from build123d import *

# Parameters (mm, degrees)
EXTRUDE_2_DEPTH     = 5
EXTRUDE_2_2_DEPTH   = 5
EXTRUDE_3_DEPTH     = 50
EXTRUDE_4_DEPTH     = 10
CUT_EXTRUDE_1_DEPTH = 7.5
SKETCH_9_R          = 1.25
CUT_EXTRUDE_3_DEPTH = 20
SKETCH_10_R         = 8
SKETCH_10_R_2       = 1.25
CUT_EXTRUDE_7_DEPTH = 5
SKETCH_1_9_R        = 1.25
EXTRUDE_5_DEPTH     = 45
SKETCH_14_R         = 1.25
CUT_EXTRUDE_8_DEPTH = 14
EXTRUDE_6_DEPTH     = 15


# Read off the part's stored shape, not the designer's step: the extrude step
with BuildPart() as part:
    # Sketch 1 → Extrude 2 (new body)
    with BuildSketch(Plane(origin=(0, 0, 0), x_dir=(1, 0, 0), z_dir=(0, 1, 0))):
        with BuildLine():
            Line((56.548408352, 75.246242124), (-83.374180902, 75.246242124))
            Line((-83.374180902, 75.246242124), (-83.374180902, 65.246242124))
            ThreePointArc((-83.374180902, 65.246242124), (-84.838646996, 61.710708218), (-88.374180902, 60.246242124))
            Line((-88.374180902, 60.246242124), (-98.374180902, 60.246242124))
            Line((-98.374180902, 60.246242124), (-98.374180902, -54.753757876))
            Line((-98.374180902, -54.753757876), (-88.374180902, -54.753757876))
            ThreePointArc((-88.374180902, -54.753757876), (-84.838646996, -56.21822397), (-83.374180902, -59.753757876))
            Line((-83.374180902, -59.753757876), (-83.374180902, -69.753757876))
            Line((-83.374180902, -69.753757876), (96.625819098, -69.753757876))
            Line((96.625819098, -69.753757876), (96.625819098, -59.753757876))
            ThreePointArc((96.625819098, -59.753757876), (98.090285193, -56.21822397), (101.625819098, -54.753757876))
            Line((101.625819098, -54.753757876), (111.625819098, -54.753757876))
            Line((111.625819098, -54.753757876), (111.625819098, 14.619924984))
            Line((111.625819098, 14.619924984), (105.067595409, 14.619924984))
            ThreePointArc((105.067595409, 14.619924984), (100.381304866, 17.876743713), (101.799973847, 23.404452606))
            Line((101.799973847, 23.404452606), (106.763929588, 27.690411234))
            Line((106.763929588, 27.690411234), (71.686518841, 68.316728374))
            Line((71.686518841, 68.316728374), (64.816029914, 62.384638559))
            ThreePointArc((64.816029914, 62.384638559), (59.467315828, 61.622843062), (56.548408352, 66.169166182))
            Line((56.548408352, 66.169166182), (56.548408352, 75.246242124))
        make_face()
        Polygon((18.529202454, 9.525154804), (27.612068748, 17.367446554), (47.217798123, -5.33971918), (38.134931829, -13.18201093), align=None, mode=Mode.SUBTRACT)
    extrude(amount=EXTRUDE_2_DEPTH)

    # Sketch 1_6 → Extrude 3 (add)
    with BuildSketch(Plane(origin=(0, 0, 0), x_dir=(1, 0, 0), z_dir=(0, 1, 0))):
        with BuildLine():
            Line((116.625819098, 34.900965901), (116.625819098, -62.253757876))
            ThreePointArc((116.625819098, -62.253757876), (112.964653863, -71.092592641), (104.125819098, -74.753757876))
            Line((104.125819098, -74.753757876), (-90.874180902, -74.753757876))
            ThreePointArc((-90.874180902, -74.753757876), (-99.713015666, -71.092592641), (-103.374180902, -62.253757876))
            Line((-103.374180902, -62.253757876), (-103.374180902, 67.746242124))
            ThreePointArc((-103.374180902, 67.746242124), (-99.713015666, 76.585076889), (-90.874180902, 80.246242124))
            Line((-90.874180902, 80.246242124), (76.449603474, 80.246242124))
            ThreePointArc((76.449603474, 80.246242124), (79.57124226, 79.565726803), (82.126394907, 77.647674468))
            Line((82.126394907, 77.647674468), (114.802610532, 39.802398244))
            ThreePointArc((114.802610532, 39.802398244), (116.155254913, 37.515737807), (116.625819098, 34.900965901))
        make_face()
        with BuildLine():
            ThreePointArc((111.625819098, 19.269608073), (111.155254913, 21.88437998), (109.802610532, 24.171040417))
            Line((109.802610532, 24.171040417), (67.947110848, 72.647674468))
            ThreePointArc((67.947110848, 72.647674468), (65.3919582, 74.565726803), (62.270319414, 75.246242124))
            Line((62.270319414, 75.246242124), (-90.874180902, 75.246242124))
            ThreePointArc((-90.874180902, 75.246242124), (-96.17748176, 73.049542983), (-98.374180902, 67.746242124))
            Line((-98.374180902, 67.746242124), (-98.374180902, -62.253757876))
            ThreePointArc((-98.374180902, -62.253757876), (-96.17748176, -67.557058735), (-90.874180902, -69.753757876))
            Line((-90.874180902, -69.753757876), (104.125819098, -69.753757876))
            ThreePointArc((104.125819098, -69.753757876), (109.429119957, -67.557058735), (111.625819098, -62.253757876))
            Line((111.625819098, -62.253757876), (111.625819098, 19.269608073))
        make_face(mode=Mode.SUBTRACT)
    extrude(amount=EXTRUDE_3_DEPTH)

    # Extrude 4 outline → Extrude 4 (add)
    with BuildSketch(Plane(origin=(0, 0, 0), x_dir=(1, 0, 0), z_dir=(0, 1, 0))):
        Polygon((43.4332705, -8.607340743), (23.827541125, 14.099824991), (22.313730076, 12.792776366), (41.919459451, -9.914389368), align=None)
    extrude(amount=EXTRUDE_4_DEPTH)

    # Sketch 6 → Cut-Extrude 1 (cut)
    with BuildSketch(Plane(origin=(85.459602861, 0, -73.787185323), x_dir=(-0.6535243124977221, 0, -0.7569055244707755), z_dir=(0.7569055244707754, 0, -0.653524312497722))):
        with BuildLine():
            Line((-22.999642003, 24.2), (-22.999642003, 21.9))
            Line((-22.999642003, 21.9), (-16.799642003, 21.9))
            Line((-16.799642003, 21.9), (-16.799642003, 24.2))
            ThreePointArc((-16.799642003, 24.2), (-15.999642003, 25), (-16.799642003, 25.8))
            Line((-16.799642003, 25.8), (-16.799642003, 27.1))
            Line((-16.799642003, 27.1), (-17.799642003, 28.1))
            Line((-17.799642003, 28.1), (-21.999642003, 28.1))
            Line((-21.999642003, 28.1), (-22.999642003, 27.1))
            Line((-22.999642003, 27.1), (-22.999642003, 25.8))
            ThreePointArc((-22.999642003, 25.8), (-23.799642003, 25), (-22.999642003, 24.2))
        make_face()
    extrude(amount=-CUT_EXTRUDE_1_DEPTH, mode=Mode.SUBTRACT)

    # Sketch 9 → Cut-Extrude 3 (cut)
    with BuildSketch(Plane(origin=(79.782811427, 0, -68.885752979), x_dir=(-0.6535243124977224, 0, -0.7569055244707754), z_dir=(0.7569055244707754, 0, -0.6535243124977224))):
        with Locations((-19.899642003, 25)):
            Circle(SKETCH_9_R)
    extrude(amount=-CUT_EXTRUDE_3_DEPTH, mode=Mode.SUBTRACT)

    # Sketch 10 → Cut-Extrude 7 (cut)
    with BuildSketch(Plane.ZY.offset(103.374180902)):
        with Locations((-2.746242124, 25)):
            Circle(SKETCH_10_R)
        with Locations((-59.046242124, 24)):
            Circle(SKETCH_10_R_2)
        with Locations((53.553757876, 24)):
            Circle(SKETCH_10_R_2)
    extrude(amount=-CUT_EXTRUDE_7_DEPTH, mode=Mode.SUBTRACT)

    # Sketch 1_9 → Extrude 5 (add)
    # profile 1 of 5: a face of its own
    with BuildSketch(Plane(origin=(0, 0, 0), x_dir=(1, 0, 0), z_dir=(0, 1, 0))):
        with BuildLine():
            Line((-83.374180902, 75.246242124), (-90.874180902, 75.246242124))
            ThreePointArc((-90.874180902, 75.246242124), (-96.17748176, 73.049542983), (-98.374180902, 67.746242124))
            Line((-98.374180902, 67.746242124), (-98.374180902, 60.246242124))
            Line((-98.374180902, 60.246242124), (-88.374180902, 60.246242124))
            ThreePointArc((-88.374180902, 60.246242124), (-84.838646996, 61.710708218), (-83.374180902, 65.246242124))
            Line((-83.374180902, 65.246242124), (-83.374180902, 75.246242124))
        make_face()
        with Locations(Location((-90.874180902, 67.746242124, 0), (0, 0, 90))):
            Circle(SKETCH_1_9_R, mode=Mode.SUBTRACT)
    # profile 2 of 5: a face of its own
    with BuildSketch(Plane(origin=(0, 0, 0), x_dir=(1, 0, 0), z_dir=(0, 1, 0))):
        with BuildLine():
            Line((-88.374180902, -54.753757876), (-98.374180902, -54.753757876))
            Line((-98.374180902, -54.753757876), (-98.374180902, -62.253757876))
            ThreePointArc((-98.374180902, -62.253757876), (-96.17748176, -67.557058735), (-90.874180902, -69.753757876))
            Line((-90.874180902, -69.753757876), (-83.374180902, -69.753757876))
            Line((-83.374180902, -69.753757876), (-83.374180902, -59.753757876))
            ThreePointArc((-83.374180902, -59.753757876), (-84.838646996, -56.21822397), (-88.374180902, -54.753757876))
        make_face()
        with Locations(Location((-90.874180902, -62.253757876, 0), (0, 0, 90))):
            Circle(SKETCH_1_9_R, mode=Mode.SUBTRACT)
    # profile 3 of 5: a face of its own
    with BuildSketch(Plane(origin=(0, 0, 0), x_dir=(1, 0, 0), z_dir=(0, 1, 0))):
        with BuildLine():
            Line((96.625819098, -59.753757876), (96.625819098, -69.753757876))
            Line((96.625819098, -69.753757876), (104.125819098, -69.753757876))
            ThreePointArc((104.125819098, -69.753757876), (109.429119957, -67.557058735), (111.625819098, -62.253757876))
            Line((111.625819098, -62.253757876), (111.625819098, -54.753757876))
            Line((111.625819098, -54.753757876), (101.625819098, -54.753757876))
            ThreePointArc((101.625819098, -54.753757876), (98.090285193, -56.21822397), (96.625819098, -59.753757876))
        make_face()
        with Locations(Location((104.125819098, -62.253757876, 0), (0, 0, 90))):
            Circle(SKETCH_1_9_R, mode=Mode.SUBTRACT)
    # profile 4 of 5: a face of its own
    with BuildSketch(Plane(origin=(0, 0, 0), x_dir=(1, 0, 0), z_dir=(0, 1, 0))):
        with BuildLine():
            Line((109.802610532, 24.171040417), (106.763929588, 27.690411234))
            Line((106.763929588, 27.690411234), (101.799973847, 23.404452606))
            ThreePointArc((101.799973847, 23.404452606), (100.381304866, 17.876743713), (105.067595409, 14.619924984))
            Line((105.067595409, 14.619924984), (111.625819098, 14.619924984))
            Line((111.625819098, 14.619924984), (111.625819098, 19.269608073))
            ThreePointArc((111.625819098, 19.269608073), (111.155254913, 21.88437998), (109.802610532, 24.171040417))
        make_face()
        with Locations(Location((105.067595409, 19.619924984, 0), (0, 0, 90))):
            Circle(SKETCH_1_9_R, mode=Mode.SUBTRACT)
    # profile 5 of 5: a face of its own
    with BuildSketch(Plane(origin=(0, 0, 0), x_dir=(1, 0, 0), z_dir=(0, 1, 0))):
        with BuildLine():
            Line((62.270319414, 75.246242124), (56.548408352, 75.246242124))
            Line((56.548408352, 75.246242124), (56.548408352, 66.169166182))
            ThreePointArc((56.548408352, 66.169166182), (59.467315828, 61.622843062), (64.816029914, 62.384638559))
            Line((64.816029914, 62.384638559), (71.686518841, 68.316728374))
            Line((71.686518841, 68.316728374), (67.947110848, 72.647674468))
            ThreePointArc((67.947110848, 72.647674468), (65.3919582, 74.565726803), (62.270319414, 75.246242124))
        make_face()
        with Locations(Location((61.548408352, 66.169166182, 0), (0, 0, 90))):
            Circle(SKETCH_1_9_R, mode=Mode.SUBTRACT)
    extrude(amount=EXTRUDE_5_DEPTH)

    # Sketch 14 → Cut-Extrude 8 (cut)
    with BuildSketch(Plane(origin=(74.862925518, 0, -64.637844948), x_dir=(0.6535243124977226, 0, 0.7569055244707751), z_dir=(-0.7569055244707751, 0, 0.6535243124977226))):
        with Locations((34.899642003, 25)):
            Circle(SKETCH_14_R)
        with Locations((4.899642003, 25)):
            Circle(SKETCH_14_R)
    extrude(amount=-CUT_EXTRUDE_8_DEPTH, mode=Mode.SUBTRACT)



with BuildPart() as body_2:
    # Sketch 1 → Extrude 2 2 (new body)
    with BuildSketch(Plane(origin=(0, 0, 0), x_dir=(1, 0, 0), z_dir=(0, 1, 0))):
        Polygon((40.165648938, -4.822813121), (27.095162688, 10.315297369), (25.581351639, 9.008248744), (38.651837889, -6.129861746), align=None)
    extrude(amount=EXTRUDE_2_2_DEPTH)


with BuildPart() as part_1:
    add(part.part)

    add(body_2.part)  # Extrude 6 merges body 2
    # Sketch 1_10 → Extrude 6 (add)
    with BuildSketch(Plane(origin=(0, 0, 0), x_dir=(1, 0, 0), z_dir=(0, 1, 0))):
        Polygon((23.827541125, 14.099824991), (27.095162688, 10.315297369), (40.165648938, -4.822813121), (43.4332705, -8.607340743), (47.217798123, -5.33971918), (27.612068748, 17.367446554), align=None)
        Polygon((38.651837889, -6.129861746), (25.581351639, 9.008248744), (22.313730076, 12.792776366), (18.529202454, 9.525154804), (38.134931829, -13.18201093), (41.919459451, -9.914389368), align=None)
    extrude(amount=EXTRUDE_6_DEPTH)


solid = part_1.part
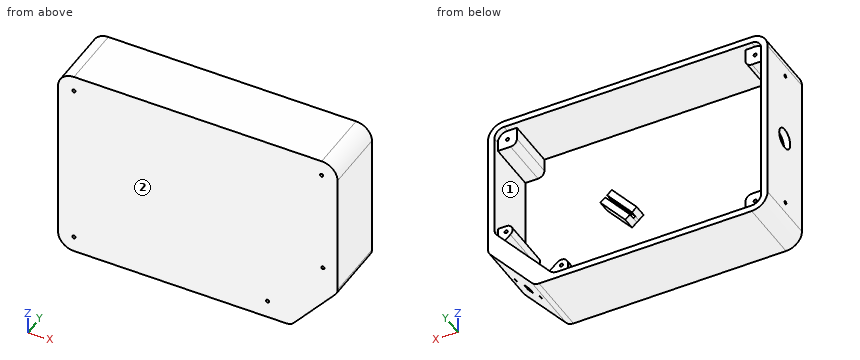
Could you check a few things on this model? Use its own coordinates, in mm. Face numbers are marked on the shaded views. A direction names the side the tool comes from. Coordinates: 2 decimals unless noted, no trailing zeros. Write each loop counter-clockwise with the first axis right and the second up, starting at its lowest first coordinate (ties: lowest second). Pieces come first, ordered by that corner, then holes. Notation, with made-up numbers: (75.5, -31) - (108.5, -31) arc R34 ccw to (108.5, 8) - close; hole circle Ø1 at (87.5, 17). An arc over 180 degrees is marked (long way). Put each result on its own line as item: value. Start each with the question number.
Q1. Please list where these lines run through material, in increasing order: L1, parallel to Z at x = -8.5, y = 16; L2, parallel to X at y = 40.5, z = 8; L3, parallel to X at y = 9, z = 12.5.
Q2. I want a section at A-A on z = -0.5. Write out the boundary of the cut face in (x, y).
Q3. I want a section at B-B on x = -79.5. Write out the boundary of the cut face in (y, z).
Q4. Which directions (+Z, -Z, +X, -X, +Y, -Y) give clear straight access to the entire face, cutting with the end or side of a thin tool? Please do the marked faces 1 and 2.
Q5. I'm going to push flat-ended pins straight in: P1, Ø3, axis at y = 18, z = 65.5, coming from the -X side; P2, Ø1.5, axis at x = 104.13, z = 62.25, coming from the -Y side; P3, Ø1, axis at x = 11.5, z = 15, coming from the -Y side; P4, Ø5, axis at x = 86, y = 34, coming from the -Z side. Where does each tip first touch, or does it pass through?
Q6. I want a section at C-C on y = 38.5. Count the separate pieces of the cut face and the enclosed holes in it, plus the area to 3 significant figures.
Checks:
1. L1: -80.25 to -75.25, 69.75 to 74.75
1. L2: -103.37 to -98.37, 111.63 to 116.63
1. L3: -103.37 to -98.37, 37.55 to 38.92, 111.63 to 116.63
2. outline: (-103.37, 0) - (116.63, 0) - (116.63, 50) - (111.63, 50) - (111.63, 5) - (42.18, 5) - (42.18, 15) - (35.57, 15) - (35.57, 10) - (32.93, 10) - (32.93, 15) - (26.32, 15) - (26.32, 5) - (-98.37, 5) - (-98.37, 17.32) - (-103.37, 17.32) - close; (-103.37, 32.68) - (-98.37, 32.68) - (-98.37, 50) - (-103.37, 50) - close
3. outline: (0, -80.25) - (50, -80.25) - (50, -75.25) - (5, -75.25) - (5, 69.75) - (50, 69.75) - (50, 74.75) - (0, 74.75) - close
4. face 1: +Y
4. face 2: +Z, -Z, +X, -X, -Y
5. P1: x = -103.25
5. P2: through
5. P3: y = 0
5. P4: z = -76.06
6. separate pieces: 1
6. enclosed holes: 6
6. area: 4,890 mm²
